from build123d import *

# Parameters (mm, degrees)
F0_R           = 29.5
F1_DEPTH       = 40
F3_D           = 10.3
F3_DEPTH       = 25
F3_TIP         = 3.094432188
F5_D           = 6.5
F5_CBORE_D     = 10
F5_CBORE_DEPTH = 23


with BuildPart() as f1:
    # F0 (on Top) → F1 (new body)
    with BuildSketch(Plane.XY):
        Circle(F0_R)
    extrude(amount=F1_DEPTH)

    # F3
    with Locations(Plane.XY.offset(40)):
        with Locations((-12.5, 0), (12.5, 0)):
            Hole(F3_D / 2, depth=F3_DEPTH)
            with Locations((0, 0, -(F3_DEPTH + F3_TIP / 2))):  # 118° drill point
                Cone(0, F3_D / 2, F3_TIP, mode=Mode.SUBTRACT)

    # F5 (through all)
    with Locations(Plane.XY.offset(40)):
        with Locations((0, 19), (0, -19)):
            CounterBoreHole(F5_D / 2, F5_CBORE_D / 2, F5_CBORE_DEPTH)


solid = f1.part
Model file for the job. Use its own axes, mm. A direction names the side the tool comes from. Round coordinates to 2 decimals unless told otherwise and drop trailing zeros. Loops run counter-clockwise (first coordinate to the right, second up) from the corner with the lowest first, then second, coordinate; pieces in that order, holes last. Notation, with made-up numbers: (10.5, 78.25) -> (37.5, 78.25) arc R24 cw to (37.5, 96.25) -> close; hole circle Ø10 at (39.5, 32). An arc over 180 degrees is marked (long way). Answer as CSV lines item,"result". Start each with the question number.
1) Probe line 1 along Y through (x, z) = (0, 23); line 2 along Y through (x, z) = (0, 13); line 3 along X through (y, z) = (23, 26). List the from-to ranges inside material, lowest first.
2) Pin check, flat tips, straight feed: P1, Ø8, axis at x = -1, y = 18.5, coming from the +Z side; P2, Ø2, axis at x = 22, y = 21.5, coming from the +Z side; P3, Ø8, axis at y = 17, z = 18.5, coming from the +X side; P4, Ø10, axis at x = -0.5, z = 15.5, coming from the +Y side. Stop position of each tip, or through.
3) Mould opens along Y. For faces 3 (the face through (11.61, 0.04, 12.44)), 4 (the face through (28.14, 8.86, 19.72)), 5 (the face through (0, 0, 0)) say: +Y half, -Y half, draft (parallel to the pull), parting line (faces both ways), or undercut.
4) Slice it at A-A (x = 0). List the corners of the cut face in (y, z).
5) Tool access for faces 1 (the face through (0, 0, 40)), 2 (the face through (-17.41, 1.55, 27.33)): list every direction of +Z, -Z, +X, -X, +Y, -Y with a clear straight run to the whole face (end or side of a thin tool).
6) Slice it at D-D (z = 33.5). List the corners of the cut face in (x, y).
7) Slice it at B-B (y = -19). List the corners of the cut face in (x, z).
8) Slice it at C-C (z = 5.5). List the corners of the cut face in (x, y), plus the area to 3 significant figures.
Filled in:
1,line 1,"y = -29.5 to -24, -14 to 14, 24 to 29.5"
1,line 2,"y = -29.5 to -22.25, -15.75 to 15.75, 22.25 to 29.5"
1,line 3,"x = -18.47 to -3, 3 to 18.47"
2,P1,"stops at z = 40"
2,P2,"passes through"
2,P3,"stops at x = 26.48"
2,P4,"stops at y = 29.5"
3,face 3,"undercut"
3,face 4,"parting line"
3,face 5,"draft"
4,outline,"(-29.5, 0) -> (-22.25, 0) -> (-22.25, 17) -> (-24, 17) -> (-24, 40) -> (-29.5, 40) -> close; (-15.75, 0) -> (15.75, 0) -> (15.75, 17) -> (14, 17) -> (14, 40) -> (-14, 40) -> (-14, 17) -> (-15.75, 17) -> close; (22.25, 0) -> (29.5, 0) -> (29.5, 40) -> (24, 40) -> (24, 17) -> (22.25, 17) -> close"
5,face 1,"+Z, +X, -X, +Y, -Y"
5,face 2,"+Z"
6,outline,"circle Ø59 at (0, 0); hole circle Ø10.3 at (-12.5, 0); hole circle Ø10 at (0, -19); hole circle Ø10 at (0, 19); hole circle Ø10.3 at (12.5, 0)"
7,outline,"(-22.57, 0) -> (-3.25, 0) -> (-3.25, 17) -> (-5, 17) -> (-5, 40) -> (-22.57, 40) -> close; (3.25, 0) -> (22.57, 0) -> (22.57, 40) -> (5, 40) -> (5, 17) -> (3.25, 17) -> close"
8,outline,"circle Ø59 at (0, 0); hole circle Ø6.5 at (0, -19); hole circle Ø6.5 at (0, 19)"
8,area,"2,670 mm2"
